Model file for the job. Use its own axes, mm. Face numbers are marked on the shaded views. A direction names the side the tool comes from. Give positions to 0.01 mm unless a question says otherwise; leave off trailing zeros. Order: outer loops, then holes, each group sorted by start corner. A loop starts at its lowest first (then second) coordinate and runs counter-clockwise, first axis right, second up. Notation, with made-up numbers: M 84,-24 L 129,-24 A23 cw 129,11 Z; hole C 68,55.5 d5. An arc over 180 degrees is marked long. Return JSON: item names as keys, results as strings. Group by question number.
1. Slice it at D-D on z = -23. List the corners of the cut face in (x, y), then the cut area to 3 significant figures.
2. Wall check: probe 1 along Y at (x, z) = (0, -4.5); probe 2 along X at (y, z) = (1.5, -18.5); probe 3 along X at (y, z) = (-1.75, -6). Give the ranges that are in metal, low to high. Write a range as [from, to].
3. 3-axis set-ups, long thin cutter, end or side, ignore diameter. For the marked faces 4 and 5: which of +Z, -Z, +X, -X, +Y, -Y reach the whole face in a straight line?
4. Pin check, flat tips, straight feed: pin 1 (1 mm diameter, centred on y = 2.5, z = -28.5, fed in from +X); pin 2 (2.5 mm diameter, centred on y = -1, z = -7.5, fed in from -X); pin 3 (4.5 mm diameter, centred on y = -2, z = -9, fed in from +X). Stop position of each tip, or through.
5. Slice it at C-C on z = -14.5. List the corners of the cut face in (x, y), then the cut area to 3 significant figures.
6. Two-plate mould, pull along X, no slides. Class the marked faces 1, 2 and 3: released by +X, released by -X, zero draft, split by the parting line, or undercut.
7. Slice it at A-A on z = -2.5. List the corners of the cut face in (x, y).
8. Slice it at B-B on x = 0. List the corners of the cut face in (y, z).
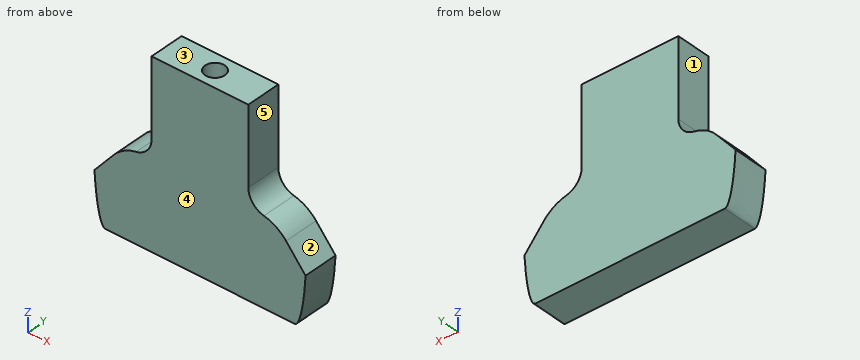
from build123d import *
from OCP.BRepFilletAPI import BRepFilletAPI_MakeChamfer

# Parameters (mm, degrees)
SKETCH2_W           = 55
SKETCH2_H           = 9
SKETCH2_R           = 2.55
BOSS_EXTRUDE1_DEPTH = 12.2
SKETCH3_W           = 55
SKETCH3_H           = 9
BOSS_EXTRUDE2_DEPTH = 35
CUT_EXTRUDE1_REACH  = 57.363
CHAMFER1_SIZE       = 8
CHAMFER1_SIZE2      = 9.534028741
FILLET1_SIZE        = 20
FILLET1_SIZE_2      = 3
FILLET2_R           = 10


with BuildPart() as part:
    # Sketch2 → Boss-Extrude1 (new body)
    with BuildSketch(Plane.XY):
        Rectangle(SKETCH2_W, SKETCH2_H)
        Circle(SKETCH2_R, mode=Mode.SUBTRACT)
    extrude(amount=-BOSS_EXTRUDE1_DEPTH)

    # Sketch3 → Boss-Extrude2 (add)
    with BuildSketch(Plane(origin=(0, 0, -12.2), x_dir=(-1, 0, 0), z_dir=(0, 0, -1))):
        Rectangle(SKETCH3_W, SKETCH3_H)
    extrude(amount=BOSS_EXTRUDE2_DEPTH)

    # Sketch5 → Cut-Extrude1 (cut, up to next)
    with BuildSketch(Plane.XZ.offset(4.5), mode=Mode.PRIVATE) as cut_extrude1_sk1:
        with BuildLine():
            Line((27.5, 0), (12.5, 0))
            Line((12.5, 0), (12.5, -20))
            ThreePointArc((12.5, -20), (13.964466094, -23.535533906), (17.5, -25))
            Line((17.5, -25), (27.5, -25))
            Line((27.5, -25), (27.5, 0))
        make_face()
    cut_extrude1_tool1 = extrude(cut_extrude1_sk1.sketch, amount=-CUT_EXTRUDE1_REACH, mode=Mode.PRIVATE) & part.part
    # Sketch5 → Cut-Extrude1 (cut, up to next)
    with BuildSketch(Plane.XZ.offset(4.5), mode=Mode.PRIVATE) as cut_extrude1_sk2:
        with BuildLine():
            Line((-12.5, 0), (-12.5, -20))
            ThreePointArc((-12.5, -20), (-13.964466094, -23.535533906), (-17.5, -25))
            Line((-17.5, -25), (-27.5, -25))
            Line((-27.5, -25), (-27.5, 0))
            Line((-27.5, 0), (-12.5, 0))
        make_face()
    cut_extrude1_tool2 = extrude(cut_extrude1_sk2.sketch, amount=-CUT_EXTRUDE1_REACH, mode=Mode.PRIVATE) & part.part
    add(cut_extrude1_tool1.solids().sort_by_distance((20.092648, -4.5, -12.33478))[0], mode=Mode.SUBTRACT)
    add(cut_extrude1_tool2.solids().sort_by_distance((-20.092648, -4.5, -12.33478))[0], mode=Mode.SUBTRACT)

    # Chamfer1: one chamfer whose edges measure the first distance from different faces: ONE call of the kernel's chamfer builder (chamfer() names one face for all edges)
    chamfer1_edges_1 = [part.edges().sort_by_distance(p)[0] for p in [
        (27.5, 0, -25),
    ]]
    chamfer1_side_1 = [part.faces().sort_by_distance(p)[0] for p in [
        (22.5, 0, -25),
    ]]
    chamfer1_edges_2 = [part.edges().sort_by_distance(p)[0] for p in [
        (-27.5, 0, -25),
    ]]
    chamfer1_side_2 = [part.faces().sort_by_distance(p)[0] for p in [
        (-22.5, 0, -25),
    ]]
    chamfer1 = BRepFilletAPI_MakeChamfer(part.part.solid().wrapped)
    for e in chamfer1_edges_1:
        chamfer1.Add(CHAMFER1_SIZE, CHAMFER1_SIZE2, e.wrapped, chamfer1_side_1[0].wrapped)  # the first distance lies on this face
    for e in chamfer1_edges_2:
        chamfer1.Add(CHAMFER1_SIZE, CHAMFER1_SIZE2, e.wrapped, chamfer1_side_2[0].wrapped)  # the first distance lies on this face
    add(Compound.cast(chamfer1.Shape()), mode=Mode.REPLACE)

    # Fillet1
    # an asymmetric fillet: 20, 3 mm, written as the material it takes off along each edge
    with BuildSketch(Plane(origin=(-27.5, -54.5, -47.2), x_dir=(0, 0, 1), z_dir=(0, 1, 0))) as fillet1_piece_1:
        with BuildLine():
            Bezier((FILLET1_SIZE, 0), (0, 0), (0, FILLET1_SIZE_2), weights=[1, 0.707106781, 1])
            Line((0, FILLET1_SIZE_2), (0, 0))
            Line((0, 0), (FILLET1_SIZE, 0))
        make_face()
    extrude(amount=109, mode=Mode.SUBTRACT)
    with BuildSketch(Plane(origin=(27.5, 54.5, -47.2), x_dir=(-1, 0, 0), z_dir=(0, -1, 0))) as fillet1_piece_2:
        with BuildLine():
            Bezier((FILLET1_SIZE_2, 0), (0, 0), (0, -FILLET1_SIZE), weights=[1, 0.707106781, 1])
            Line((0, -FILLET1_SIZE), (0, 0))
            Line((0, 0), (FILLET1_SIZE_2, 0))
        make_face()
    extrude(amount=109, mode=Mode.SUBTRACT)

    # Fillet2
    fillet2_edges = [part.edges().sort_by_distance(p)[0] for p in [
        (19.5, 0, -25),
        (-19.5, 0, -25),
    ]]
    fillet(fillet2_edges, radius=FILLET2_R)


solid = part.part
Result:
{
 "1": {"outline": "M -13.5,-4.5 L 13.5,-4.5 L 13.5,4.5 L -13.5,4.5 Z", "area": "243 mm2"},
 "2": {"probe 1": "y = [-4.5, -2.55], [2.55, 4.5]", "probe 2": "x = [-12.5, 12.5]", "probe 3": "x = [-12.5, -1.85], [1.85, 12.5]"},
 "3": {"face 4": "+Z, -Z, +X, -X, -Y", "face 5": "+Z, +X, +Y, -Y"},
 "4": {"pin 1": "stops at x = 22.86", "pin 2": "stops at x = -12.5", "pin 3": "stops at x = 12.5"},
 "5": {"outline": "M -12.5,-4.5 L 12.5,-4.5 L 12.5,4.5 L -12.5,4.5 Z", "area": "225 mm2"},
 "6": {"face 1": "released by -X", "face 2": "released by +X", "face 3": "zero draft"},
 "7": {"outline": "M -12.5,-4.5 L 12.5,-4.5 L 12.5,4.5 L -12.5,4.5 Z; hole C 0,0 d5.1"},
 "8": {"outline": "M -4.5,-47.2 L 4.5,-47.2 L 4.5,0 L 2.55,0 L 2.55,-12.2 L -2.55,-12.2 L -2.55,0 L -4.5,0 Z"}
}
